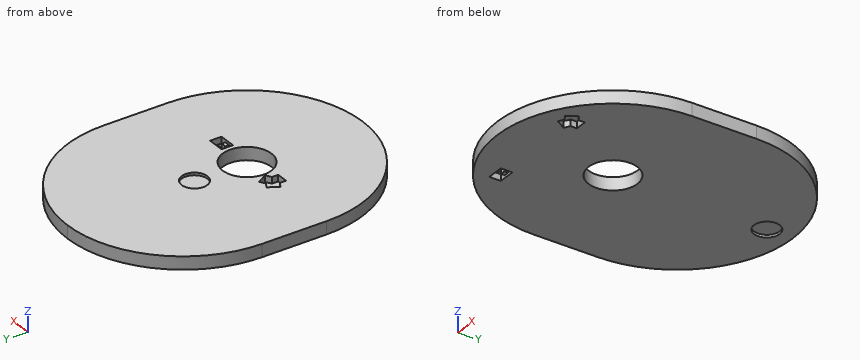
```python
from build123d import *

# Parameters (mm, degrees)
F1_DEPTH  = 5
F3_DEPTH  = 2.5
F4_W      = 6.5
F4_H      = 4.5
F5_DEPTH  = 2.5
F6_W      = 2
F6_H      = 1.5
F7_DEPTH  = 1.5
F8_R      = 5
F9_DEPTH  = 1
F10_R     = 9.5
F11_DEPTH = 10
F14_DEPTH = 2.5
F12_R     = 5
F15_DEPTH = 1
F16_W     = 6.5
F16_H     = 4.5
F17_DEPTH = 2.5
F18_W     = 2
F18_H     = 1.5
F19_DEPTH = 1.5
F20_R     = 44.99999


# Not quite as in the source:
# - a fillet or chamfer is up to 0.001 mm smaller than in the source, because OpenCascade refuses the exact size


with BuildPart() as f1:
    # F0 (on Top) → F1 (new body)
    with BuildSketch(Plane.XY):
        with BuildLine():
            Line((-45, 70), (-45, 0))
            ThreePointArc((-45, 0), (0, -45), (45, 0))
            Line((45, 0), (45, 70))
            Line((45, 70), (-45, 70))
        make_face()
    extrude(amount=F1_DEPTH)

    # F2 (on face) → F3 (cut)
    with BuildSketch(Plane.XY.offset(5)):
        Polygon((-14.5, 2.6008529611), (-16.625, 3.8277222831), (-18.875, -0.0693920339), (-16.75, -1.2962613559), (-16.75, -3.75), (-12.25, -3.75), (-12.25, -1.2962613559), (-10.125, -0.0693920339), (-12.375, 3.8277222831), align=None)
    extrude(amount=-F3_DEPTH, mode=Mode.SUBTRACT)

    # F4 (on face) → F5 (cut)
    with BuildSketch(Plane.XY.offset(5)):
        with Locations((14.5, 0)):
            Rectangle(F4_W, F4_H)
    extrude(amount=-F5_DEPTH, mode=Mode.SUBTRACT)

    # F6 (on face) → F7 (join)
    with BuildSketch(Plane.XY.offset(2.5)):
        with Locations((14.5, 1.5)):
            Rectangle(F6_W, F6_H)
        with Locations((14.5, -1.5)):
            Rectangle(F6_W, F6_H)
    extrude(amount=F7_DEPTH)

    # F8 (on face) → F9 (cut)
    with BuildSketch(Plane.XY.offset(5)):
        with Locations((0, 20.4880452948)):
            Circle(F8_R)
    extrude(amount=-F9_DEPTH, mode=Mode.SUBTRACT)

    # F10 (on face) → F11 (cut)
    with BuildSketch(Plane(origin=(0, 0, 0), x_dir=(1, 0, 0), z_dir=(0, 0, -1))):
        Circle(F10_R)
    extrude(amount=-F11_DEPTH, mode=Mode.SUBTRACT)

    # F13 (on face) → F14 (cut)
    with BuildSketch(Plane(origin=(0, 0, 0), x_dir=(1, 0, 0), z_dir=(0, 0, -1))):
        Polygon((20, 32.6008529611), (17.875, 33.8277222831), (15.625, 29.9306079661), (17.75, 28.7037386441), (17.75, 26.25), (22.25, 26.25), (22.25, 28.7037386441), (24.375, 29.9306079661), (22.125, 33.8277222831), align=None)
    extrude(amount=-F14_DEPTH, mode=Mode.SUBTRACT)

    # F12 (on face) → F15 (cut)
    with BuildSketch(Plane(origin=(0, 0, 0), x_dir=(1, 0, 0), z_dir=(0, 0, -1))):
        with Locations((0, -60)):
            Circle(F12_R)
    extrude(amount=-F15_DEPTH, mode=Mode.SUBTRACT)

    # F16 (on face) → F17 (cut)
    with BuildSketch(Plane(origin=(0, 0, 0), x_dir=(1, 0, 0), z_dir=(0, 0, -1))):
        with Locations((-20, 30)):
            Rectangle(F16_W, F16_H)
    extrude(amount=-F17_DEPTH, mode=Mode.SUBTRACT)

    # F18 (on face) → F19 (join)
    with BuildSketch(Plane(origin=(0, 0, 2.5), x_dir=(1, 0, 0), z_dir=(0, 0, -1))):
        with Locations((-20, 31.5)):
            Rectangle(F18_W, F18_H)
        with Locations((-20, 28.5)):
            Rectangle(F18_W, F18_H)
    extrude(amount=F19_DEPTH)

    # F20 (radius 45 in the source; OpenCascade refuses exactly that, so slightly less here)
    f20_edges = [f1.edges().sort_by_distance(p)[0] for p in [
        (-45, 70, 2.5),
        (45, 70, 2.5),
    ]]
    fillet(f20_edges, radius=F20_R)


solid = f1.part
```
Can you work these out from the model? Positions are in its coordinate system, mm. Coordinates: 2 decimals unless noted, no trailing zeros. Loops run counter-clockwise (first coordinate to the right, second up) from the corner with the lowest first, then second, coordinate; pieces in that order, holes last.
1) For pin 1 (1.2 mm diameter, centred on y = -28.5, z = 2, fed in from +X); pin 2 (1.2 mm diameter, centred on x = -20, z = 2, fed in from +Y); pin 3 (1 mm diameter, centred on y = 50.5, z = 4.5, fed in from -X); pin 4 (15 mm diameter, centred on x = 0, y = 0, fed in from +Z), each with a flat end and sliding along its axis, tell me the tip position at first contact or that it passes through.
2) I need wall thicknesses on probe 1 along X at (y, z) = (-29, 0.45); probe 2 along X at (y, z) = (0, 1.3); probe 3 along X at (y, z) = (25.5, 3.6). Which ranges of each line are inside material? Lowest first, please.
3) Imagine slicing it at B-B on x = -36. List the corners of the cut face in (y, z) for me.
4) Imagine slicing it at C-C on y = 60. List the corners of the cut face in (x, z) for me.
5) Imagine slicing it at A-A on y = 5.5. List the corners of the cut face in (x, z) for me, plus the area to 3 significant figures.
6) Imagine slicing it at D-D on x = 38. List the corners of the cut face in (y, z) for me.
Completed:
1. pin 1: stops at x = 35.31
1. pin 2: stops at y = 65.6
1. pin 3: stops at x = -37.42
1. pin 4: passes through
2. probe 1: x = -34.41 to -23.25, -16.75 to 17.24, 22.76 to 34.41
2. probe 2: x = -45 to -9.5, 9.5 to 45
2. probe 3: x = -45 to 45
3. outline: (-27, 0) - (52, 0) - (52, 5) - (-27, 5) - close
4. outline: (-28.28, 0) - (-5, 0) - (-5, 1) - (5, 1) - (5, 0) - (28.28, 0) - (28.28, 5) - (-28.28, 5) - close
5. outline: (-45, 0) - (-7.75, 0) - (-7.75, 5) - (-45, 5) - close; (7.75, 0) - (45, 0) - (45, 5) - (7.75, 5) - close
5. area: 373 mm2
6. outline: (-24.1, 0) - (49.1, 0) - (49.1, 5) - (-24.1, 5) - close
